Design review of the part shown in the three views and the two pictorial views. Dimensions are in mm from the part's minimum x, y and z. A direction names the side the tool comes from. Give positions to 0.01 mm unless a question says otherwise; leave off trailing zeros. Loops run counter-clockwise (first coordinate to the right, second up) from the corner with the lowest first, then second, coordinate; pieces in that order, holes last.
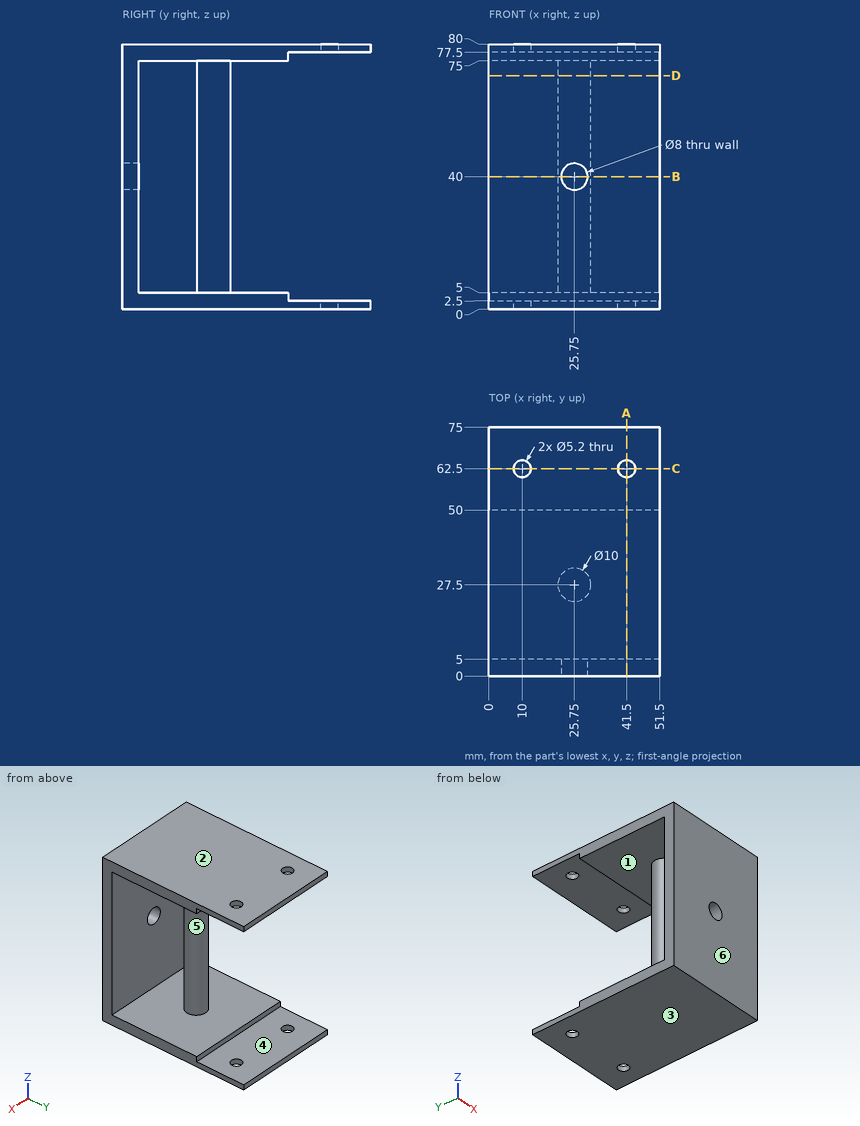
Q1. Draft analysis for pull direction Z (two halves, no side actions). For the marked faces 1, 2 and 3, state which applies: pulls with the +Z half, pulls with the -Z half, needs draft (parallel to the pull), parting line crosses it, or undercut.
Results:
face 1: undercut
face 2: pulls with the +Z half
face 3: pulls with the -Z half
Q2. Insertion check: pin 1 (12 mm diameter, centred on y = 23.5, z = 61.5, fed in from -X); pin 2 (9 mm diameter, centred on x = 25.75, z = 40, fed in from +Y); pin 3 (5 mm diameter, centred on x = 25, z = 39, fed in from -Y). Each pin has a flat end and moves straight along its axis. Give the tip position at first contact, or say it passes through.
Results:
pin 1: stops at x = 20.75
pin 2: stops at y = 32.5
pin 3: stops at y = 22.5
Q3. Take a section at A-A (x = 41.5). Give the boundary of the cut face in (y, z), plus the area to 3 significant figures.
Results:
outline: (0, 0) - (59.9, 0) - (59.9, 2.5) - (50, 2.5) - (50, 5) - (5, 5) - (5, 75) - (50, 75) - (50, 77.5) - (59.9, 77.5) - (59.9, 80) - (0, 80) - close; (65.1, 0) - (75, 0) - (75, 2.5) - (65.1, 2.5) - close; (65.1, 77.5) - (75, 77.5) - (75, 80) - (65.1, 80) - close
area: 949 mm2
Q4. Tool access review of the marked faces 4, 5 and 6: name each direction out of +Z, -Z, +X, -X, +Y, -Y from which nothing blocks a thin tool from reaching the whole face with its end or side.
Results:
face 4: +X, -X, +Y
face 5: none
face 6: +Z, -Z, +X, -X, -Y
Q5. Take a section at D-D (z = 70.5). Give the boundary of the cut face in (x, y).
Results:
outline: (0, 0) - (51.5, 0) - (51.5, 5) - (0, 5) - close; circle Ø10 at (25.75, 27.5)
Q6. Take a section at B-B (z = 40). Give the boundary of the cut face in (x, y).
Results:
outline: (0, 0) - (21.75, 0) - (21.75, 5) - (0, 5) - close; circle Ø10 at (25.75, 27.5); (29.75, 0) - (51.5, 0) - (51.5, 5) - (29.75, 5) - close
Q7. Take a section at C-C (y = 62.5). Give the boundary of the cut face in (x, z).
Results:
outline: (0, 0) - (7.4, 0) - (7.4, 2.5) - (0, 2.5) - close; (0, 77.5) - (7.4, 77.5) - (7.4, 80) - (0, 80) - close; (12.6, 0) - (38.9, 0) - (38.9, 2.5) - (12.6, 2.5) - close; (12.6, 77.5) - (38.9, 77.5) - (38.9, 80) - (12.6, 80) - close; (44.1, 0) - (51.5, 0) - (51.5, 2.5) - (44.1, 2.5) - close; (44.1, 77.5) - (51.5, 77.5) - (51.5, 80) - (44.1, 80) - close
Q8. Wall thickness on line 1 (Z direction, x = 3.5, y = 5.5); line 2 (Y direction, x = 41.5, z = 0.7); line 3 (Z direction, x = 21, y = 55.5): over which ranges is each line inside the solid? List them lowest first.
Results:
line 1: z = 0 to 5, 75 to 80
line 2: y = 0 to 59.9, 65.1 to 75
line 3: z = 0 to 2.5, 77.5 to 80
